Verification items for the finished model (mm, model axes). A direction names the side the tool comes from. Give positions to 0.01 mm unless a question says otherwise; leave off trailing zeros. Loops run counter-clockwise (first coordinate to the right, second up) from the corner with the lowest first, then second, coordinate; pieces in that order, holes last. Notation, with made-up numbers: (35, 65.5) -> (71, 65.5) arc R29 ccw to (71, 87.5) -> close; hole circle Ø7 at (-11, 63.25). An arc over 180 degrees is marked (long way). Answer in a Markdown table with one row per item. Add a question column.
Q1. Release check for a two-part mould opening along Y. For faces 5 (the face through (-3, -14, 12)), 6 (the face through (-3, -19, 2)), 7 (the face through (-4, -7, 1)), 8 (the face through (-1, 18, 11)) record: pulls with the +Y half, pulls with the -Y half, needs draft (parallel to the pull), parting line crosses it, or undercut.
Q2. Material ranges on probe 1 along Y at (x, z) = (-8.75, 16.5); probe 2 along X at (y, z) = (3, 12.75); probe 3 along Z at (x, y) = (-4, 18.5), recorded low to high.
Q3. Section check D-D on x = -2. Enter the section's corners in (y, z).
Q4. Gauge pin test, flat ends, axial feed: P1, Ø10, axis at x = -1, z = 16.5, coming from the -Y side; P2, Ø2.5, axis at y = -19.5, z = 9.5, coming from the +X side; P3, Ø5, axis at x = -6.5, z = 11, coming from the -Y side. Record the tip position at first contact, or that the pin passes through.
Q5. Section check C-C on z = 15.5. Enter the section's corners in (x, y), and give its area (3 significant figures).
Q6. Section check A-A on x = -5. Enter the section's corners in (y, z), and give its area (3 significant figures).
Q7. Section check B-B on y = 20. Enter the section's corners in (x, z).
Q8. Set-up check for faces 1 (the face through (3, 0, 1)), 2 (the face through (-2.5, -16, 8)), 3 (the face through (0.5, -16, 8)), 4 (the face through (3.3, -0.2, 2)): record each of +Z, -Z, +X, -X, +Y, -Y from which the full face is reachable in a straight line by a thin tool's end or side.
```python
from build123d import *

# Parameters (mm, degrees)
SKETCH_2_W          = 22
SKETCH_2_H          = 28
EXTRUDE_1_DEPTH     = 22
SKETCH_3_W          = 18
SKETCH_3_H          = 24
CUT_EXTRUDE_1_DEPTH = 20
SKETCH_4_W          = 14
SKETCH_4_H          = 14
CUT_EXTRUDE_3_DEPTH = 27.776855678
SKETCH_6_W          = 20
SKETCH_6_H          = 24
CUT_EXTRUDE_4_DEPTH = 5
SKETCH_7_W          = 22
SKETCH_7_H          = 2
EXTRUDE_3_DEPTH     = 10
SKETCH_8_W          = 22
SKETCH_8_H          = 2
EXTRUDE_4_DEPTH     = 10
RIB_3_REACH         = 36.699
SKETCH_10_WALL_W    = 91.095121896
SKETCH_10_WALL_H    = 3
RIB_4_REACH         = 36.699
SKETCH_11_WALL_W    = 91.095121896
SKETCH_11_WALL_H    = 3
FILLET_1_R          = 3


with BuildPart() as part:
    # ｽｹｯﾁ2 → ﾎﾞｽ - 押し出し1 (new body)
    with BuildSketch(Plane.XY):
        Rectangle(SKETCH_2_W, SKETCH_2_H)
    extrude(amount=EXTRUDE_1_DEPTH)

    # ｽｹｯﾁ3 → ｶｯﾄ - 押し出し1 (cut)
    with BuildSketch(Plane.XY.offset(22)):
        Rectangle(SKETCH_3_W, SKETCH_3_H)
    extrude(amount=-CUT_EXTRUDE_1_DEPTH, mode=Mode.SUBTRACT)

    # ｽｹｯﾁ4 → ｶｯﾄ - 押し出し3 (cut, through all)
    with BuildSketch(Plane.XY.offset(2)):
        with Locations((-4, 0)):
            Rectangle(SKETCH_4_W, SKETCH_4_H)
    extrude(amount=-CUT_EXTRUDE_3_DEPTH, mode=Mode.SUBTRACT)

    # ｽｹｯﾁ6 → ｶｯﾄ - 押し出し4 (cut)
    with BuildSketch(Plane.ZY.offset(11)):
        with Locations((12, 0)):
            Rectangle(SKETCH_6_W, SKETCH_6_H)
    extrude(amount=-CUT_EXTRUDE_4_DEPTH, mode=Mode.SUBTRACT)

    # ｽｹｯﾁ7 → ﾎﾞｽ - 押し出し3 (add)
    with BuildSketch(Plane.XZ.offset(14)):
        with Locations((0, 1)):
            Rectangle(SKETCH_7_W, SKETCH_7_H)
    extrude(amount=EXTRUDE_3_DEPTH)

    # ｽｹｯﾁ8 → ﾎﾞｽ - 押し出し4 (add)
    with BuildSketch(Plane(origin=(0, 14, 0), x_dir=(1, 0, 0), z_dir=(0, 1, 0))):
        with Locations((0, -1)):
            Rectangle(SKETCH_8_W, SKETCH_8_H)
    extrude(amount=EXTRUDE_4_DEPTH)

    # ｽｹｯﾁ10 wall → ﾘﾌﾞ3 (add, up to next)
    with BuildSketch(Plane(origin=(-1, -18, 11), x_dir=(0, -0.406138466053, -0.91381154862), z_dir=(0, 0.91381154862, -0.406138466053)), mode=Mode.PRIVATE) as rib_3_sk1:
        Rectangle(SKETCH_10_WALL_W, SKETCH_10_WALL_H)
    rib_3_tool1 = extrude(rib_3_sk1.sketch, amount=RIB_3_REACH, mode=Mode.PRIVATE) - part.part
    add(rib_3_tool1.solids().sort_by_distance((-1, -18, 11))[0])

    # ｽｹｯﾁ11 wall → ﾘﾌﾞ4 (add, up to next)
    with BuildSketch(Plane(origin=(-1, 18, 11), x_dir=(0, 0.406138466053, -0.91381154862), z_dir=(0, 0.91381154862, 0.406138466053)), mode=Mode.PRIVATE) as rib_4_sk1:
        Rectangle(SKETCH_11_WALL_W, SKETCH_11_WALL_H)
    rib_4_tool1 = extrude(rib_4_sk1.sketch, amount=-RIB_4_REACH, mode=Mode.PRIVATE) - part.part
    add(rib_4_tool1.solids().sort_by_distance((-1, 18, 11))[0])

    # ﾌｨﾚｯﾄ1
    fillet_1_edges = [part.edges().sort_by_distance(p)[0] for p in [
        (-11, 13, 22),
        (-11, -13, 22),
    ]]
    fillet(fillet_1_edges, radius=FILLET_1_R)


solid = part.part
```
Taken from the geometry:
| question | item | result |
|---|---|---|
| 1 | face 5 | pulls with the -Y half |
| 1 | face 6 | needs draft |
| 1 | face 7 | undercut |
| 1 | face 8 | pulls with the +Y half |
| 2 | probe 1 | y = -14 to -12, 12 to 14 |
| 2 | probe 2 | x = 9 to 11 |
| 2 | probe 3 | z = 0 to 2 |
| 3 | outline | (-24, 0) -> (-7, 0) -> (-7, 2) -> (-12, 2) -> (-12, 22) -> (-14, 22) -> (-14, 20) -> (-22, 2) -> (-24, 2) -> close; (7, 0) -> (24, 0) -> (24, 2) -> (22, 2) -> (14, 20) -> (14, 22) -> (12, 22) -> (12, 2) -> (7, 2) -> close |
| 4 | P1 | stops at y = -17.78 |
| 4 | P2 | stops at x = 0.5 |
| 4 | P3 | stops at y = -14 |
| 5 | outline | (-11, -14) -> (-2.5, -14) -> (-2.5, -16) -> (0.5, -16) -> (0.5, -14) -> (11, -14) -> (11, 14) -> (0.5, 14) -> (0.5, 16) -> (-2.5, 16) -> (-2.5, 14) -> (-11, 14) -> (-11, 12) -> (9, 12) -> (9, -12) -> (-11, -12) -> close |
| 5 | area | 148 mm² |
| 6 | outline | (-24, 0) -> (-7, 0) -> (-7, 2) -> (-12, 2) -> (-12, 22) -> (-14, 22) -> (-14, 2) -> (-24, 2) -> close; (7, 0) -> (24, 0) -> (24, 2) -> (14, 2) -> (14, 22) -> (12, 22) -> (12, 2) -> (7, 2) -> close |
| 6 | area | 148 mm² |
| 7 | outline | (-11, 0) -> (11, 0) -> (11, 2) -> (0.5, 2) -> (0.5, 6.5) -> (-2.5, 6.5) -> (-2.5, 2) -> (-11, 2) -> close |
| 8 | face 1 | +Z, -Z, -X |
| 8 | face 2 | +Z, -X, -Y |
| 8 | face 3 | +Z, +X, -Y |
| 8 | face 4 | +Z, -X |
